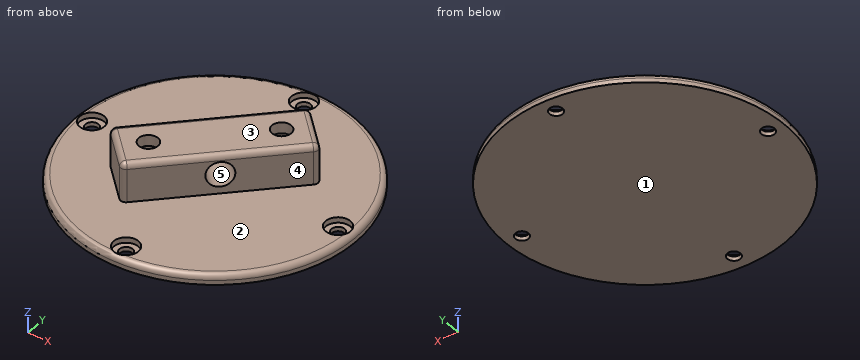
```python
from build123d import *

# Parameters (mm, degrees)
F0_R         = 25.5
F0_R_2       = 1.2
F1_DEPTH     = 1.8
F2_R         = 2.25
F3_DEPTH     = 1
F4_R         = 1.75
F5_DEPTH     = 7
F6_START     = 2
F6_DEPTH     = 3
F7_R         = 2.25
F8_DEPTH     = 41.0634458405
F9_T1_DEPTH  = 6
F9_T3_DEPTH  = 8
F9_T5_DEPTH  = 28
F9_T7_DEPTH  = 28
F9_T9_DEPTH  = 8
F9_S13_W     = 1
F9_S13_H     = 1
F9_T14_DEPTH = 1
F9_T20_DEPTH = 1
F9_S25_W     = 1
F9_S25_H     = 1
F9_T26_DEPTH = 1
F9_T32_DEPTH = 1


# Not quite as in the source:
# - a fillet or chamfer that OpenCascade refuses, or shapes differently, is made with other operations: its cross-section is extruded or revolved along the edge and cut away or added


with BuildPart() as f1:
    # F0 (on Top) → F1 (new body)
    with BuildSketch(Plane.XY):
        Circle(F0_R)
        with Locations((0, -22.5)):
            Circle(F0_R_2, mode=Mode.SUBTRACT)
        with Locations((-22.5, 0)):
            Circle(F0_R_2, mode=Mode.SUBTRACT)
        with Locations((22.5, 0)):
            Circle(F0_R_2, mode=Mode.SUBTRACT)
        with Locations((0, 22.5)):
            Circle(F0_R_2, mode=Mode.SUBTRACT)
    extrude(amount=F1_DEPTH)

    # F2 (on face) → F3 (cut)
    with BuildSketch(Plane.XY.offset(1.8)):
        with Locations((0, -22.5)):
            Circle(F2_R)
        with Locations((-22.5, 0)):
            Circle(F2_R)
        with Locations((0, 22.5)):
            Circle(F2_R)
        with Locations((22.5, 0)):
            Circle(F2_R)
    extrude(amount=-F3_DEPTH, mode=Mode.SUBTRACT)

    # F4 (on face) → F5 (join)
    with BuildSketch(Plane.XY.offset(1.8)):
        Polygon((7.0710678119, 14.1421356237), (-14.1421356237, -7.0710678119), (-7.0710678119, -14.1421356237), (14.1421356237, 7.0710678119), align=None)
        Polygon((-6.1744923397, -10.4171330268), (-9.5205575546, -9.5205575546), (-10.4171330268, -6.1744923397), (-7.967643284, -3.7250025969), (-4.6215780691, -4.6215780691), (-3.7250025969, -7.967643284), align=None, mode=Mode.SUBTRACT)
        Polygon((3.7250025969, 7.967643284), (6.1744923397, 10.4171330268), (9.5205575546, 9.5205575546), (10.4171330268, 6.1744923397), (7.967643284, 3.7250025969), (4.6215780691, 4.6215780691), align=None, mode=Mode.SUBTRACT)
        Polygon((-10.4171330268, -6.1744923397), (-9.5205575546, -9.5205575546), (-6.1744923397, -10.4171330268), (-3.7250025969, -7.967643284), (-4.6215780691, -4.6215780691), (-7.967643284, -3.7250025969), align=None)
        with Locations((-7.0710678119, -7.0710678119)):
            Circle(F4_R, mode=Mode.SUBTRACT)
        Polygon((9.5205575546, 9.5205575546), (6.1744923397, 10.4171330268), (3.7250025969, 7.967643284), (4.6215780691, 4.6215780691), (7.967643284, 3.7250025969), (10.4171330268, 6.1744923397), align=None)
        with Locations((7.0710678119, 7.0710678119)):
            Circle(F4_R, mode=Mode.SUBTRACT)
    extrude(amount=F5_DEPTH)

    # F4 (on face) → F6 (cut)
    with BuildSketch(Plane.XY.offset(1.8).offset(F6_START)):
        Polygon((-10.4171330268, -6.1744923397), (-9.5205575546, -9.5205575546), (-6.1744923397, -10.4171330268), (-3.7250025969, -7.967643284), (-4.6215780691, -4.6215780691), (-7.967643284, -3.7250025969), align=None)
        with Locations((-7.0710678119, -7.0710678119)):
            Circle(F4_R, mode=Mode.SUBTRACT)
        Polygon((9.5205575546, 9.5205575546), (6.1744923397, 10.4171330268), (3.7250025969, 7.967643284), (4.6215780691, 4.6215780691), (7.967643284, 3.7250025969), (10.4171330268, 6.1744923397), align=None)
        with Locations((7.0710678119, 7.0710678119)):
            Circle(F4_R, mode=Mode.SUBTRACT)
    extrude(amount=F6_DEPTH, mode=Mode.SUBTRACT)

    # F7 (on face) → F8 (cut, through all)
    with BuildSketch(Plane(origin=(-3.5355339059, 3.5355339059, 0), x_dir=(-0.7071067812, -0.7071067812, 0), z_dir=(-0.7071067812, 0.7071067812, 0))):
        with Locations((0, 5.3)):
            Circle(F7_R)
    extrude(amount=-F8_DEPTH, mode=Mode.SUBTRACT)

    # F9: fillet of radius 1 on 9 edges, made by hand

    # F9_s2 → F9_t1 (cut)
    with BuildSketch(Plane.XY.offset(1.8)):
        with BuildLine():
            ThreePointArc((-13.4350288425, -6.3639610307), (-13.7279220614, -7.0710678119), (-13.4350288425, -7.7781745931))
            Line((-13.4350288425, -7.7781745931), (-14.1421356237, -7.0710678119))
            Line((-14.1421356237, -7.0710678119), (-13.4350288425, -6.3639610307))
        make_face()
        with BuildLine():
            ThreePointArc((-7.7781745931, -13.4350288425), (-7.0710678119, -13.7279220614), (-6.3639610307, -13.4350288425))
            Line((-6.3639610307, -13.4350288425), (-7.0710678119, -14.1421356237))
            Line((-7.0710678119, -14.1421356237), (-7.7781745931, -13.4350288425))
        make_face()
        with BuildLine():
            ThreePointArc((13.4350288425, 6.3639610307), (13.7279220614, 7.0710678119), (13.4350288425, 7.7781745931))
            Line((13.4350288425, 7.7781745931), (14.1421356237, 7.0710678119))
            Line((14.1421356237, 7.0710678119), (13.4350288425, 6.3639610307))
        make_face()
        with BuildLine():
            ThreePointArc((6.3639610307, 13.4350288425), (7.0710678119, 13.7279220614), (7.7781745931, 13.4350288425))
            Line((7.7781745931, 13.4350288425), (7.0710678119, 14.1421356237))
            Line((7.0710678119, 14.1421356237), (6.3639610307, 13.4350288425))
        make_face()
    extrude(amount=F9_T1_DEPTH, mode=Mode.SUBTRACT)

    # F9_s4 → F9_t3 (cut)
    with BuildSketch(Plane(origin=(-2.8284271247, 2.8284271247, 0), x_dir=(0, 0, 1), z_dir=(0.7071067812, -0.7071067812, 0))):
        with BuildLine():
            ThreePointArc((7.8, 15), (8.5071067812, 14.7071067812), (8.8, 14))
            Line((8.8, 14), (8.8, 15))
            Line((8.8, 15), (7.8, 15))
        make_face()
    extrude(amount=F9_T3_DEPTH, mode=Mode.SUBTRACT)

    # F9_s6 → F9_t5 (cut)
    with BuildSketch(Plane(origin=(9.8994949366, 9.8994949366, 0), x_dir=(0, 0, 1), z_dir=(-0.7071067812, -0.7071067812, 0))):
        with BuildLine():
            ThreePointArc((7.8, 5), (8.5071067812, 4.7071067812), (8.8, 4))
            Line((8.8, 4), (8.8, 5))
            Line((8.8, 5), (7.8, 5))
        make_face()
    extrude(amount=F9_T5_DEPTH, mode=Mode.SUBTRACT)

    # F9_s8 → F9_t7 (cut)
    with BuildSketch(Plane(origin=(-9.8994949366, -9.8994949366, 0), x_dir=(0, 0, 1), z_dir=(0.7071067812, 0.7071067812, 0))):
        with BuildLine():
            ThreePointArc((7.8, 5), (8.5071067812, 4.7071067812), (8.8, 4))
            Line((8.8, 4), (8.8, 5))
            Line((8.8, 5), (7.8, 5))
        make_face()
    extrude(amount=F9_T7_DEPTH, mode=Mode.SUBTRACT)

    # F9_s10 → F9_t9 (cut)
    with BuildSketch(Plane(origin=(2.8284271247, -2.8284271247, 0), x_dir=(0, 0, 1), z_dir=(-0.7071067812, 0.7071067812, 0))):
        with BuildLine():
            ThreePointArc((7.8, 15), (8.5071067812, 14.7071067812), (8.8, 14))
            Line((8.8, 14), (8.8, 15))
            Line((8.8, 15), (7.8, 15))
        make_face()
    extrude(amount=F9_T9_DEPTH, mode=Mode.SUBTRACT)


with BuildPart() as f9_tool12:
    # F9_s13 → F9_t14 (new body)
    with BuildSketch(Plane(origin=(-2.8284271247, 2.8284271247, 0), x_dir=(0, 0, 1), z_dir=(-0.7071067812, 0.7071067812, 0))):
        with Locations((8.3, -14.5)):
            Rectangle(F9_S13_W, F9_S13_H)
    extrude(amount=F9_T14_DEPTH)

    # F9_s15 → F9_t16 (revolve, cut)
    with BuildSketch(Plane(origin=(-12.7279220614, -7.0710678119, 7.8), x_dir=(0.5, 0.5, -0.7071067812), z_dir=(0.5, 0.5, 0.7071067812))):
        with BuildLine():
            ThreePointArc((0, -1), (1, 0), (0, 1))
            Line((0, 1), (0, -1))
        make_face()
    revolve(axis=Axis((-12.7279220614, -7.0710678119, 7.8), (-0.7071067812, 0.7071067812, 0)), mode=Mode.SUBTRACT)


with BuildPart() as f1_1:
    add(f1.part)

    # F9_t11: cut F9_tool12
    add(f9_tool12.part, mode=Mode.SUBTRACT)


with BuildPart() as f9_tool18:
    # F9_s19 → F9_t20 (new body)
    with BuildSketch(Plane.XY.offset(7.8)):
        Polygon((-7.0710678119, -12.7279220614), (-7.7781745931, -13.4350288425), (-7.0710678119, -14.1421356237), (-6.3639610307, -13.4350288425), align=None)
    extrude(amount=F9_T20_DEPTH)

    # F9_s21 → F9_t22 (revolve, cut)
    with BuildSketch(Plane(origin=(-7.0710678119, -12.7279220614, 7.8), x_dir=(0, 1, 0), z_dir=(1, 0, 0))):
        with BuildLine():
            ThreePointArc((0, -1), (1, 0), (0, 1))
            Line((0, 1), (0, -1))
        make_face()
    revolve(axis=Axis((-7.0710678119, -12.7279220614, 7.8), (0, 0, 1)), mode=Mode.SUBTRACT)


with BuildPart() as f1_2:
    add(f1_1.part)

    # F9_t17: cut F9_tool18
    add(f9_tool18.part, mode=Mode.SUBTRACT)


with BuildPart() as f9_tool24:
    # F9_s25 → F9_t26 (new body)
    with BuildSketch(Plane(origin=(-2.8284271247, 2.8284271247, 0), x_dir=(0, 0, 1), z_dir=(-0.7071067812, 0.7071067812, 0))):
        with Locations((8.3, 14.5)):
            Rectangle(F9_S25_W, F9_S25_H)
    extrude(amount=F9_T26_DEPTH)

    # F9_s27 → F9_t28 (revolve, cut)
    with BuildSketch(Plane(origin=(7.0710678119, 12.7279220614, 7.8), x_dir=(-0.5, -0.5, -0.7071067812), z_dir=(0.5, 0.5, -0.7071067812))):
        with BuildLine():
            ThreePointArc((0, -1), (1, 0), (0, 1))
            Line((0, 1), (0, -1))
        make_face()
    revolve(axis=Axis((7.0710678119, 12.7279220614, 7.8), (-0.7071067812, 0.7071067812, 0)), mode=Mode.SUBTRACT)


with BuildPart() as f1_3:
    add(f1_2.part)

    # F9_t23: cut F9_tool24
    add(f9_tool24.part, mode=Mode.SUBTRACT)


with BuildPart() as f9_tool30:
    # F9_s31 → F9_t32 (new body)
    with BuildSketch(Plane.XY.offset(7.8)):
        Polygon((12.7279220614, 7.0710678119), (13.4350288425, 6.3639610307), (14.1421356237, 7.0710678119), (13.4350288425, 7.7781745931), align=None)
    extrude(amount=F9_T32_DEPTH)

    # F9_s33 → F9_t34 (revolve, cut)
    with BuildSketch(Plane(origin=(12.7279220614, 7.0710678119, 7.8), x_dir=(-1, 0, 0), z_dir=(0, 1, 0))):
        with BuildLine():
            ThreePointArc((0, -1), (1, 0), (0, 1))
            Line((0, 1), (0, -1))
        make_face()
    revolve(axis=Axis((12.7279220614, 7.0710678119, 7.8), (0, 0, 1)), mode=Mode.SUBTRACT)


with BuildPart() as f1_4:
    add(f1_3.part)

    # F9_t29: cut F9_tool30
    add(f9_tool30.part, mode=Mode.SUBTRACT)

    # F9_s35 → F9_t36 (revolve, cut)
    with BuildSketch(Plane.XZ):
        with BuildLine():
            ThreePointArc((25.5, 0.8), (25.2071067812, 1.5071067812), (24.5, 1.8))
            Line((24.5, 1.8), (25.5, 1.8))
            Line((25.5, 1.8), (25.5, 0.8))
        make_face()
    revolve(axis=Axis((0, 0, 1.8), (0, 0, 1)), mode=Mode.SUBTRACT)


solid = f1_4.part
```
Part model, mm, in its own coordinate system. Face numbers are marked on the shaded views. A direction names the side the tool comes from. Coordinates: 2 decimals unless noted, no trailing zeros. Order: outer loops, then holes, each group sorted by start corner. A loop starts at its lowest first (then second) coordinate and runs counter-clockwise, first axis right, second up. Notation, with made-up numbers: (-13, 7) -> (22, 7) arc R20 cw to (22, 14) -> close; hole circle Ø8 at (58.5, -1). An arc over 180 degrees is marked (long way). Put each result on its own line as item: value. Start each with the question number.
(1) Band-saw the part on A-A (z = 6). Give the cut face in (x, y) (1 decimal), then the cut area to 3 significant figures.
(2) Band-saw the part on B-B (y = 0). Count the separate pieces of the cut face and the enclosed holes in it, then the cut area to 3 significant figures.
(3) Pin check, flat tips, straight feed: pin 1 Ø5 at (x, z) = (8.5, 7.5) entering from +Y; pin 2 Ø1.5 at (x, z) = (4.5, 6) entering from -Y; pin 3 Ø1.9 at (x, y) = (0, 22.5) entering from -Z; pin 4 Ø12 at (x, y) = (15, -14.5) entering from +Z. Stop position of each tip, or through.
(4) Which spindle directions (+Z, -Z, +X, -X, +Y, -Y) get a long thin tool onto all of the face, cutting with end or side? Do the marked faces 1 and 2. Say none if no direction does.
(5) Probe line 1 along Y through (x, z) = (0, 0.45); line 2 along Z through (x, y) = (-10, -6); line 3 along Z through (x, y) = (7, -10). List the from-to ranges inside material, lowest first. Write a range as [from, to].
(6) Mould opens along X. For the marked faces 3, 4 and 5 say: pulls with the +X half, pulls with the -X half, needs draft (parallel to the pull), parting line crosses it, or undercut.
Determined:
1. outline: (-13.4, -7.8) -> (-7.8, -13.4) arc R1 ccw to (-6.4, -13.4) -> (2, -5) -> (-5, 2) -> (-13.4, -6.4) arc R1 ccw to start; (-2, 5) -> (5, -2) -> (13.4, 6.4) arc R1 ccw to (13.4, 7.8) -> (7.8, 13.4) arc R1 ccw to (6.4, 13.4) -> close; hole (-10.4, -6.2) -> (-9.5, -9.5) -> (-6.2, -10.4) -> (-3.7, -8) -> (-4.6, -4.6) -> (-8, -3.7) -> close; hole (3.7, 8) -> (4.6, 4.6) -> (8, 3.7) -> (10.4, 6.2) -> (9.5, 9.5) -> (6.2, 10.4) -> close
1. area: 194 mm²
2. separate pieces: 3
2. enclosed holes: 1
2. area: 154 mm²
3. pin 1: stops at y = 13.73
3. pin 2: stops at y = -2.29
3. pin 3: passes through
3. pin 4: stops at z = 1.8
4. face 1: -Z, +X, -X, +Y, -Y
4. face 2: +Z
5. line 1: y = [-25.5, -23.7], [-21.3, 21.3], [23.7, 25.5]
5. line 2: z = [0, 3.8], [6.8, 8.8]
5. line 3: z = [0, 1.8]
6. face 3: needs draft
6. face 4: pulls with the +X half
6. face 5: undercut
